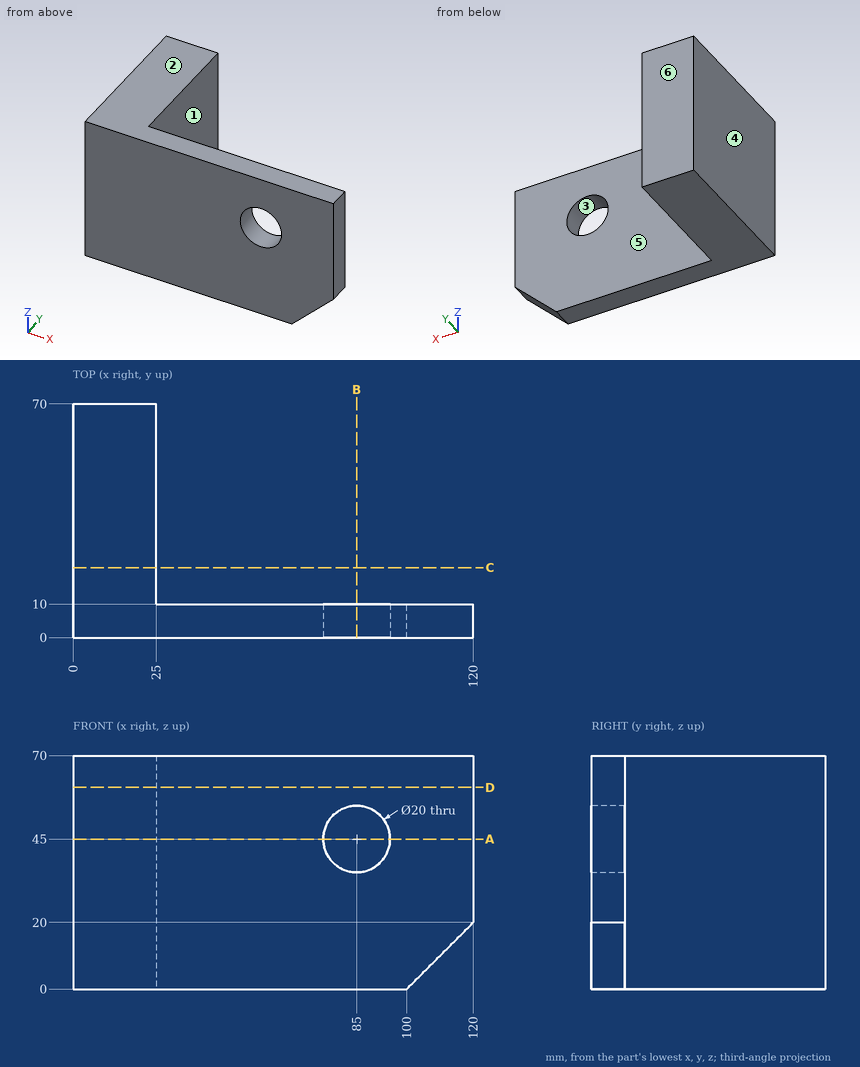
Job drawing, mm, ordinate dimensions from the low corner. One solid piece. A direction names the side the tool comes from. Coordinates: 2 decimals unless noted, no trailing zeros. Order: outer loops, then holes, each group sorted by start corner. A loop starts at its lowest first (then second) coordinate and runs counter-clockwise, first axis right, second up. Notation, with made-up numbers: (55.5, -15) -> (84.5, -15) arc R10 cw to (84.5, 4) -> close; hole circle Ø2 at (-37, 74.25). An arc over 180 degrees is marked (long way). Answer in a Markdown table with one row per item. Add a question column.
Q1. Drop flat-ended pins along their axis: pin 1 (5 mm diameter, centred on y = 47, z = 42.5, fed in from +X); pin 2 (1 mm diameter, centred on x = 80.5, z = 19.5, fed in from +Y); pin 3 (4 mm diameter, centred on y = 30, z = 17.5, fed in from -X). Give the stop position or say it passes through.
Q2. Which spindle directions (+Z, -Z, +X, -X, +Y, -Y) get a long thin tool onto all of the face, cutting with end or side? Do the marked faces 5 and 6. Say none if no direction does.
Q3. Band-saw the part on C-C, the plane y = 21. List the corners of the cut face in (x, z).
Q4. Band-saw the part on D-D, the plane z = 60.5. List the corners of the cut face in (x, y), then the cut area to 3 significant figures.
Q5. Mould opens along X. For the marked faces 1, 2, 3 and 4 say: +X half, -X half, draft (parallel to the pull), parting line (faces both ways), or undercut.
Q6. Wall check: line 1 along Z through (x, y) = (85, 2.75); line 2 along X through (y, z) = (3.5, 45); line 3 along Y through (x, z) = (57.5, 52.5). Give the ranges that are in metal, low to high. Write a range as [from, to].
Q7. Band-saw the part on A-A, the plane z = 45. List the corners of the cut face in (x, y), then the cut area to 3 significant figures.
Q8. Band-saw the part on B-B, the plane x = 85. List the corners of the cut face in (y, z).
Answers follow:
| question | item | result |
|---|---|---|
| 1 | pin 1 | x = 25 |
| 1 | pin 2 | y = 10 |
| 1 | pin 3 | x = 0 |
| 2 | face 5 | +Z, -Z, +X, +Y |
| 2 | face 6 | +Z, -Z, +X, -X, +Y |
| 3 | outline | (0, 0) -> (25, 0) -> (25, 70) -> (0, 70) -> close |
| 4 | outline | (0, 0) -> (120, 0) -> (120, 10) -> (25, 10) -> (25, 70) -> (0, 70) -> close |
| 4 | area | 2,700 mm^2 |
| 5 | face 1 | +X half |
| 5 | face 2 | draft |
| 5 | face 3 | undercut |
| 5 | face 4 | -X half |
| 6 | line 1 | [0, 35], [55, 70] |
| 6 | line 2 | [0, 75], [95, 120] |
| 6 | line 3 | [0, 10] |
| 7 | outline | (0, 0) -> (75, 0) -> (75, 10) -> (25, 10) -> (25, 70) -> (0, 70) -> close; (95, 0) -> (120, 0) -> (120, 10) -> (95, 10) -> close |
| 7 | area | 2,500 mm^2 |
| 8 | outline | (0, 0) -> (10, 0) -> (10, 35) -> (0, 35) -> close; (0, 55) -> (10, 55) -> (10, 70) -> (0, 70) -> close |
